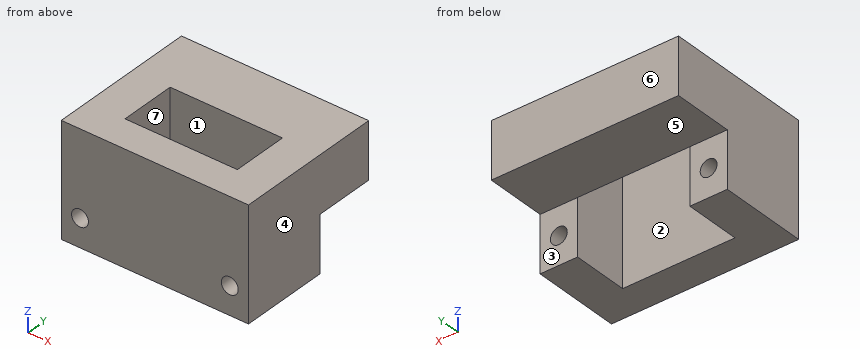
from build123d import *

# Parameters (mm, degrees)
SKETCH_1_W          = 100
SKETCH_1_H          = 80
EXTRUDE_1_DEPTH     = 15
SKETCH_4_W          = 100
SKETCH_4_H          = 47.5
EXTRUDE_2_DEPTH     = 30
SKETCH_2_W          = 60
SKETCH_2_H          = 30
CUT_EXTRUDE_1_DEPTH = 54.5
SKETCH_5_R          = 4.5
CUT_EXTRUDE_2_DEPTH = 105.522724802


with BuildPart() as part:
    # 草图1 → 凸台-拉伸1 (new, symmetric)
    with BuildSketch(Plane.XY):
        Rectangle(SKETCH_1_W, SKETCH_1_H)
    extrude(amount=EXTRUDE_1_DEPTH, both=True)

    # 草图4 → 凸台-拉伸2 (add)
    with BuildSketch(Plane.XY.offset(-15)):
        with Locations((0, -16.25)):
            Rectangle(SKETCH_4_W, SKETCH_4_H)
    extrude(amount=-EXTRUDE_2_DEPTH)

    # 草图2 → 切除-拉伸1 (cut, symmetric)
    with BuildSketch(Plane(origin=(0, 0, -15), x_dir=(-1, 0, 0), z_dir=(0, 0, -1))):
        with Locations((0, -7.5)):
            Rectangle(SKETCH_2_W, SKETCH_2_H)
    extrude(amount=CUT_EXTRUDE_1_DEPTH, both=True, mode=Mode.SUBTRACT)

    # 草图5 → 切除-拉伸2 (cut, through all)
    with BuildSketch(Plane.XZ.offset(40)):
        with Locations(Location((-40, -30, 0), (0, 0, 270))):
            Circle(SKETCH_5_R)
        with Locations(Location((40, -30, 0), (0, 0, 270))):
            Circle(SKETCH_5_R)
    extrude(amount=-CUT_EXTRUDE_2_DEPTH, mode=Mode.SUBTRACT)


solid = part.part
The listing builds one solid part. Answer for the finished solid, in the listing's coordinates (mm). Face numbers are marked on the shaded views. A direction names the side the tool comes from. Round coordinates to 2 decimals unless told otherwise and drop trailing zeros. Loops run counter-clockwise (first coordinate to the right, second up) from the corner with the lowest first, then second, coordinate; pieces in that order, holes last. Notation, with made-up numbers: M 72,-32.75 L 119,-32.75 A23 ccw 119,6.25 Z; hole C -10.75,-33.5 d5. An arc over 180 degrees is marked long. Return JSON: item names as keys, results as strings.
Q1. Find section B-B, the plane z = -30. Determine the outline of the cut face in (x, y).
Results list:
{"outline": "M -50,-40 L -44.5,-40 L -44.5,7.5 L -50,7.5 Z; M -35.5,-40 L 35.5,-40 L 35.5,7.5 L 30,7.5 L 30,-22.5 L -30,-22.5 L -30,7.5 L -35.5,7.5 Z; M 44.5,-40 L 50,-40 L 50,7.5 L 44.5,7.5 Z"}
Q2. Find the intervals of material crossed by line 1 along X through (y, z) = (-15, -30); line 2 along X through (y, z) = (-19, -16); line 3 along X through (y, z) = (-32, -29), in increasing order. Write a range as from..to.
Results list:
{"line 1": "x = -50..-44.5, -35.5..-30, 30..35.5, 44.5..50", "line 2": "x = -50..-30, 30..50", "line 3": "x = -50..-44.39, -35.61..35.61, 44.39..50"}
Q3. Each of these flat-tipped pins is pushed along its axis until it touches: pin 1 Ø12 at (x, z) = (-8.5, -30) entering from +Y; pin 2 Ø6 at (x, z) = (-42, -25.5) entering from +Y; pin 3 Ø10 at (x, y) = (21.5, 25.5) entering from -Z. Where does it stop, or does it pass through?
Results list:
{"pin 1": "stops at y = -22.5", "pin 2": "stops at y = 7.5", "pin 3": "stops at z = -15"}
Q4. Which of the six approach directions +Z, -Z, +X, -X, +Y, -Y give full straight-line access (tool end or side, diameter ignored) to the marked faces 5, 6 and 7?
Results list:
{"face 5": "-Z, +X, -X, +Y", "face 6": "+Z, -Z, +X, -X, +Y", "face 7": "+Z, -Z"}
Q5. Find section A-A, the plane y = -4. Determine the outline of the cut face in (x, z).
Results list:
{"outline": "M -50,-45 L -30,-45 L -30,15 L -50,15 Z; M 30,-45 L 50,-45 L 50,15 L 30,15 Z; hole C -40,-30 d9; hole C 40,-30 d9"}
Q6. The mould has two halves that part along X. Classify the marked faces 1, 2, 3 and 4: released by +X, released by -X, zero draft, split by the parting line, or undercut.
Results list:
{"face 1": "undercut", "face 2": "undercut", "face 3": "zero draft", "face 4": "released by +X"}
Q7. Find section C-C, the plane x = 10. Determine the outline of the cut face in (y, z).
Results list:
{"outline": "M -40,-45 L -22.5,-45 L -22.5,15 L -40,15 Z; M 7.5,-15 L 40,-15 L 40,15 L 7.5,15 Z"}
Q8. Find section D-D, the plane z = 6. Determine the outline of the cut face in (x, y).
Results list:
{"outline": "M -50,-40 L 50,-40 L 50,40 L -50,40 Z; hole M -30,-22.5 L 30,-22.5 L 30,7.5 L -30,7.5 Z"}
